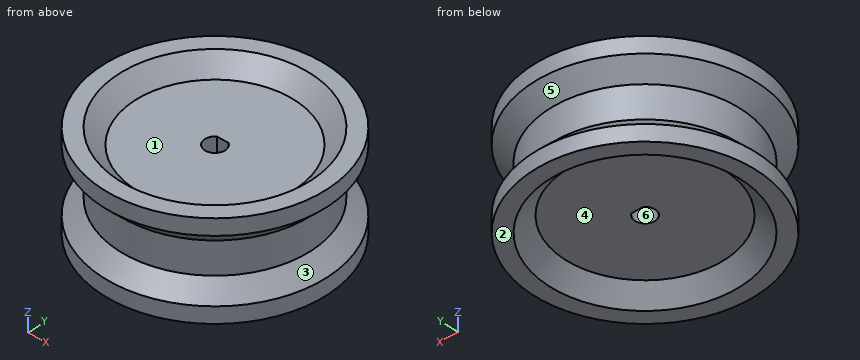
```python
from build123d import *

# Parameters (mm, degrees)
SKETCH1_R           = 35
BOSS_EXTRUDE1_DEPTH = 30
SKETCH3_R           = 25
CUT_EXTRUDE1_DEPTH  = 5
CUT_EXTRUDE2_START  = -5
SKETCH4_R           = 25
CUT_EXTRUDE2_DEPTH  = 5
CUT_EXTRUDE3_DEPTH  = 39
CHAMFER2_SIZE       = 5


with BuildPart() as part:
    # Sketch1 → Boss-Extrude1 (new body)
    with BuildSketch(Plane.XY):
        Circle(SKETCH1_R)
    extrude(amount=BOSS_EXTRUDE1_DEPTH)

    # Sketch3 → Cut-Extrude1 (cut)
    with BuildSketch(Plane.XY.offset(30)):
        Circle(SKETCH3_R)
    extrude(amount=-CUT_EXTRUDE1_DEPTH, mode=Mode.SUBTRACT)

    # Sketch4 → Cut-Extrude2 (cut)
    with BuildSketch(Plane(origin=(0, 0, 0), x_dir=(-1, 0, 0), z_dir=(0, 0, -1)).offset(CUT_EXTRUDE2_START)):
        with Locations(Location((0, 0, 0), (0, 0, 180))):
            Circle(SKETCH4_R)
    extrude(amount=CUT_EXTRUDE2_DEPTH, mode=Mode.SUBTRACT)

    # Sketch5 → Cut-Revolve1 (revolve, cut)
    with BuildSketch(Plane(origin=(0, 0, 0), x_dir=(0, 0, -1), z_dir=(1, 0, 0)), mode=Mode.PRIVATE) as cut_revolve1_sk:
        Polygon((-25, 35), (-20, 30), (-10, 30), (-5, 35), align=None)
    revolve(cut_revolve1_sk.sketch.rotate(Axis((0, 0, 49.767686579), (0, 0, -1)), 90), axis=Axis((0, 0, 49.767686579), (0, 0, -1)), mode=Mode.SUBTRACT)

    # Sketch6 → Cut-Extrude3 (cut)
    with BuildSketch(Plane.XY.offset(25)):
        with BuildLine():
            Line((-1.78605711, 2.625), (1.78605711, 2.625))
            ThreePointArc((1.78605711, 2.625), (0, -3.175), (-1.78605711, 2.625))
        make_face()
    extrude(amount=-CUT_EXTRUDE3_DEPTH, mode=Mode.SUBTRACT)

    # Chamfer2
    chamfer2_edges = [part.edges().sort_by_distance(p)[0] for p in [
        (-25, 0, 0),
        (-25, 0, 30),
    ]]
    chamfer(chamfer2_edges, length=CHAMFER2_SIZE - 0.0001)  # a hair under: the kernel refuses the full size


solid = part.part
```
The listing builds one solid part. Answer for the finished solid, in the listing's coordinates (mm). Face numbers are marked on the shaded views. A direction names the side the tool comes from. Round coordinates to 2 decimals unless told otherwise and drop trailing zeros. Loops run counter-clockwise (first coordinate to the right, second up) from the corner with the lowest first, then second, coordinate; pieces in that order, holes last. Notation, with made-up numbers: (47.25, 70.5) - (99.25, 70.5) arc R37 ccw to (99.25, 109.5) - close; hole circle Ø2 at (-19.75, 10). An arc over 180 degrees is marked (long way). Use one line per item in the form item = value. Start each with the question number.
1. The part is cut by section C-C on z = 2. Determine the outline of the cut face in (x, y).
2. For a pull along Z with two mould halves and no side action, classify the marked faces 1, 2 and 3 as pulls with the +Z half, pulls with the -Z half, needs draft (parallel to the pull), parting line crosses it, or undercut.
3. Given pin 1 Ø8 at (y, z) = (-23.5, 15.5) entering from -X; pin 2 Ø6 at (y, z) = (-22.5, 8) entering from -X; pin 3 Ø5.5 at (x, y) = (0, 0) entering from -Z; pin 4 Ø12 at (x, y) = (24, 4) entering from +Z, each flat-ended and moving along its own axis, determine where each tip first touches the part or whether it passes through.
4. The part is cut by section D-D on z = 13.5. Determine the outline of the cut face in (x, y) (3 decimals).
5. A tool of negligible diameter and unlimited length cuts with its end or side. For the marked faces 4, 5 and 6, from which of +Z, -Z, +X, -X, +Y, -Y can it reach the whole face along a straight path? Write none if from no direction.
6. Consider line 1 (Y direction, x = 0, z = 19) (3 decimals); line 2 (X direction, y = -15.5, z = 4.5); line 3 (Z direction, x = 16.5, y = 5). Determine where each line is inside the solid, lowest interval first. Write a range as [from, to].
Geometry check:
q1.outline = circle Ø70 at (0, 0); hole circle Ø56 at (0, 0)
q2.face_1 = pulls with the +Z half
q2.face_2 = pulls with the -Z half
q2.face_3 = undercut
q3.pin_1 = -22.8
q3.pin_2 = -27.5
q3.pin_3 = 5
q3.pin_4 = 30
q4.outline = circle Ø60 at (0, 0); hole (-1.786, 2.625) arc R3.175 ccw (long way) to (1.786, 2.625) - close
q5.face_4 = -Z
q5.face_5 = none
q5.face_6 = +Z, -Z
q6.line_1 = [-30, -3.175], [2.625, 30]
q6.line_2 = [-31.38, -20.25], [20.25, 31.38]
q6.line_3 = [5, 25]
